Read the model definition and answer for the solid it produces. Units are mm, in the model's axes. Face numbers are marked on the shaded views. A direction names the side the tool comes from. Give positions to 0.01 mm unless a question says otherwise; leave off trailing zeros. Loops run counter-clockwise (first coordinate to the right, second up) from the corner with the lowest first, then second, coordinate; pieces in that order, holes last.
(1) Straight lines are drawn through the part: probe 1 along Z at (x, y) = (-166, -1); probe 2 along Z at (x, y) = (-58, 1); probe 3 along X at (y, z) = (-15, -10.5). For each, find the intervals that lie inside material, in ascending order.
(2) Find section B-B, the plane x = -47.5. Write down the section's boundary in (y, z).
(3) Find section A-A, the plane x = -167. Write down the section's boundary in (y, z), then the cut area to 3 significant figures.
(4) Which of the six approach directions +Z, -Z, +X, -X, +Y, -Y give full straight-line access (tool end or side, diameter ignored) to the marked faces 1 and 2?
(5) Each of these flat-tipped pins is pushed along its axis until it touches: P1, Ø5, axis at x = -61, z = 3.5, coming from the +Y side; P2, Ø2, axis at y = -12, z = -4, coming from the -X side; P3, Ø6, axis at y = 4.5, z = -5.5, coming from the -X side. Where does it stop, or does it pass through?
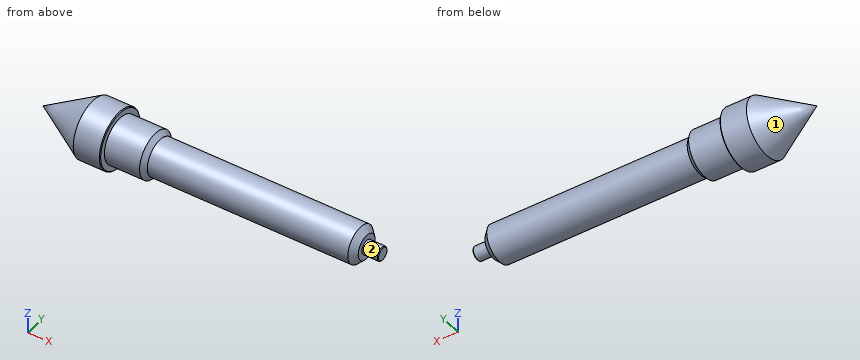
```python
from build123d import *

# Parameters (mm, degrees)
SZKIC5_R                    = 4.5
DODANIE_WYCI_GNI_CIE4_DEPTH = 10.5
SFAZOWANIE1_SIZE            = 0.5
SZKIC6_R                    = 12
DODANIE_WYCI_GNI_CIE5_DEPTH = 135
SFAZOWANIE2_SIZE            = 4
SZKIC7_R                    = 15
DODANIE_WYCI_GNI_CIE6_DEPTH = 26
SFAZOWANIE4_SIZE            = 3
SZKIC8_R                    = 19
DODANIE_WYCI_GNI_CIE7_DEPTH = 17.59
SFAZOWANIE5_SIZE            = 0.5


with BuildPart() as part:
    # Szkic5 → Dodanie-wyciągnięcie4 (new body)
    with BuildSketch(Plane(origin=(0, 0, 0), x_dir=(0, 0, -1), z_dir=(1, 0, 0))):
        with Locations(Location((0, 0, 0), (0, 0, 180))):
            Circle(SZKIC5_R)
    extrude(amount=DODANIE_WYCI_GNI_CIE4_DEPTH)

    # Sfazowanie1
    sfazowanie1_edges = [part.edges().sort_by_distance(p)[0] for p in [
        (10.5, 0, -4.5),
    ]]
    chamfer(sfazowanie1_edges, length=SFAZOWANIE1_SIZE)

    # Szkic6 → Dodanie-wyciągnięcie5 (add)
    with BuildSketch(Plane.ZY):
        Circle(SZKIC6_R)
    extrude(amount=DODANIE_WYCI_GNI_CIE5_DEPTH)

    # Sfazowanie2
    sfazowanie2_edges = [part.edges().sort_by_distance(p)[0] for p in [
        (0, 0, -12),
    ]]
    chamfer(sfazowanie2_edges, length=SFAZOWANIE2_SIZE)

    # Szkic7 → Dodanie-wyciągnięcie6 (add)
    with BuildSketch(Plane.ZY.offset(135)):
        with Locations(Location((0, 0, 0), (0, 0, 180))):
            Circle(SZKIC7_R)
    extrude(amount=DODANIE_WYCI_GNI_CIE6_DEPTH)

    # Sfazowanie4
    sfazowanie4_edges = [part.edges().sort_by_distance(p)[0] for p in [
        (-135, 0, 15),
    ]]
    chamfer(sfazowanie4_edges, length=SFAZOWANIE4_SIZE - 0.0001)  # a hair under: the kernel refuses the full size

    # Szkic8 → Dodanie-wyciągnięcie7 (add)
    with BuildSketch(Plane.ZY.offset(161)):
        with Locations(Location((0, 0, 0), (0, 0, 180))):
            Circle(SZKIC8_R)
    extrude(amount=DODANIE_WYCI_GNI_CIE7_DEPTH)

    # Szkic10 → Obrót1 (revolve)
    with BuildSketch(Plane.XY):
        Polygon((-211.498965344, 0), (-178.59, 19), (-178.59, 0), align=None)
    revolve(axis=Axis((-178.59, 0, 0), (-1, 0, 0)))

    # Sfazowanie5
    sfazowanie5_edges = [part.edges().sort_by_distance(p)[0] for p in [
        (-161, 0, 19),
    ]]
    chamfer(sfazowanie5_edges, length=SFAZOWANIE5_SIZE)


solid = part.part
```
Entries:
1. probe 1: z = -18.97 to 18.97
1. probe 2: z = -11.96 to 11.96
1. probe 3: x = -179.79 to -161
2. outline: circle Ø24 at (0, 0)
3. outline: circle Ø38 at (0, 0)
3. area: 1,130 mm2
4. face 1: -X
4. face 2: +X
5. P1: stops at y = 11.96
5. P2: stops at x = -191.32
5. P3: stops at x = -204.39
